Geometry check sheet. Reference: the model listing, model coordinates, mm. A direction names the side the tool comes from. Round coordinates to 2 decimals unless told otherwise and drop trailing zeros. Write each loop counter-clockwise with the first axis right and the second up, starting at its lowest first coordinate (ties: lowest second). Pieces come first, ordered by that corner, then holes. Notation, with made-up numbers: (-28.75, 37) - (11.25, 37) arc R7 ccw to (11.25, 49) - close; hole circle Ø6 at (21, 4). An arc over 180 degrees is marked (long way). One line per question, with ' | ' between items. Start each with the question number.
from build123d import *

# Parameters (mm, degrees)
SKETCH_1_W          = 74
SKETCH_1_H          = 24
EXTRUDE_1_DEPTH     = 400
SKETCH_2_W          = 51.146480438
SKETCH_2_H          = 44.035025014
CUT_EXTRUDE_1_DEPTH = 401


with BuildPart() as part:
    # Эскиз1 → Вытянуть-Тонкостенный1 (new body)
    with BuildSketch(Plane(origin=(0, 0, 0), x_dir=(1, 0, 0), z_dir=(0, 1, 0))):
        with BuildLine():
            Line((40, 12), (40, -12))
            ThreePointArc((40, -12), (39.121320344, -14.121320344), (37, -15))
            Line((37, -15), (-37, -15))
            ThreePointArc((-37, -15), (-39.121320344, -14.121320344), (-40, -12))
            Line((-40, -12), (-40, 12))
            ThreePointArc((-40, 12), (-39.121320344, 14.121320344), (-37, 15))
            Line((-37, 15), (37, 15))
            ThreePointArc((37, 15), (39.121320344, 14.121320344), (40, 12))
        make_face()
        Rectangle(SKETCH_1_W, SKETCH_1_H, mode=Mode.SUBTRACT)
    extrude(amount=EXTRUDE_1_DEPTH)

    # Эскиз2 → Вырез-Вытянуть1 (cut, through all)
    with BuildSketch(Plane(origin=(0, 400, 0), x_dir=(1, 0, 0), z_dir=(0, 1, 0))):
        with Locations((15.573240219, -1.044738789)):
            Rectangle(SKETCH_2_W, SKETCH_2_H)
    extrude(amount=-CUT_EXTRUDE_1_DEPTH, mode=Mode.SUBTRACT)


solid = part.part
Q1. Go/stop test with a flat-tipped pin: P1, Ø2, axis at y = 255, z = 0.5, coming from the +X side. Record where the tip stops, or that it passes through.
Q2. Section check B-B, the plane y = 49. Record the cut outline in (x, z).
Q3. Thickness scan on line 1 (Z direction, x = -28.25, y = 322); line 2 (X direction, y = 72.5, z = -0.5); line 3 (X direction, y = 131.5, z = -12.5). Record the ranges inside material, lowest first.
Q4. Section check A-A, the plane x = -16.5. Record the cut outline in (y, z).
Q5. Section check C-C, the plane z = -4. Record the cut outline in (x, y), then the cut area to 3 significant figures.
Q6. Set-up check for faces 1 (the flat face through (-24, 197, 12)), 2 (the flat face through (-37.2, 0, -0.1)): record each of +Z, -Z, +X, -X, +Y, -Y from which the full face is reachable in a straight line by a thin tool's end or side.
Result sheet:
1) P1: x = -37
2) outline: (-40, -12) arc R3 ccw to (-37, -15) - (-10, -15) - (-10, -12) - (-37, -12) - (-37, 12) - (-10, 12) - (-10, 15) - (-37, 15) arc R3 ccw to (-40, 12) - close
3) line 1: -15 to -12, 12 to 15 | line 2: -40 to -37 | line 3: -39.96 to -10
4) outline: (0, -15) - (400, -15) - (400, -12) - (0, -12) - close; (0, 12) - (400, 12) - (400, 15) - (0, 15) - close
5) outline: (-40, 0) - (-37, 0) - (-37, 400) - (-40, 400) - close | area: 1,200 mm²
6) face 1: +X, +Y, -Y | face 2: +Z, -Z, +X, -X, -Y
